Source: three-view drawing plus pictorial views. Frame: mm from the lowest corner of the part. A direction names the side the tool comes from. Coordinates: 2 decimals unless noted, no trailing zeros. Write each loop counter-clockwise with the first axis right and the second up, starting at its lowest first coordinate (ties: lowest second). Pieces come first, ordered by that corner, then holes. Notation, with made-up numbers: M 78,53 L 113,53 A21 ccw 113,74 Z; hole C 24,35.5 d9. An arc over 180 degrees is marked long. Use CSV: the item, a comma, the result in double quotes.
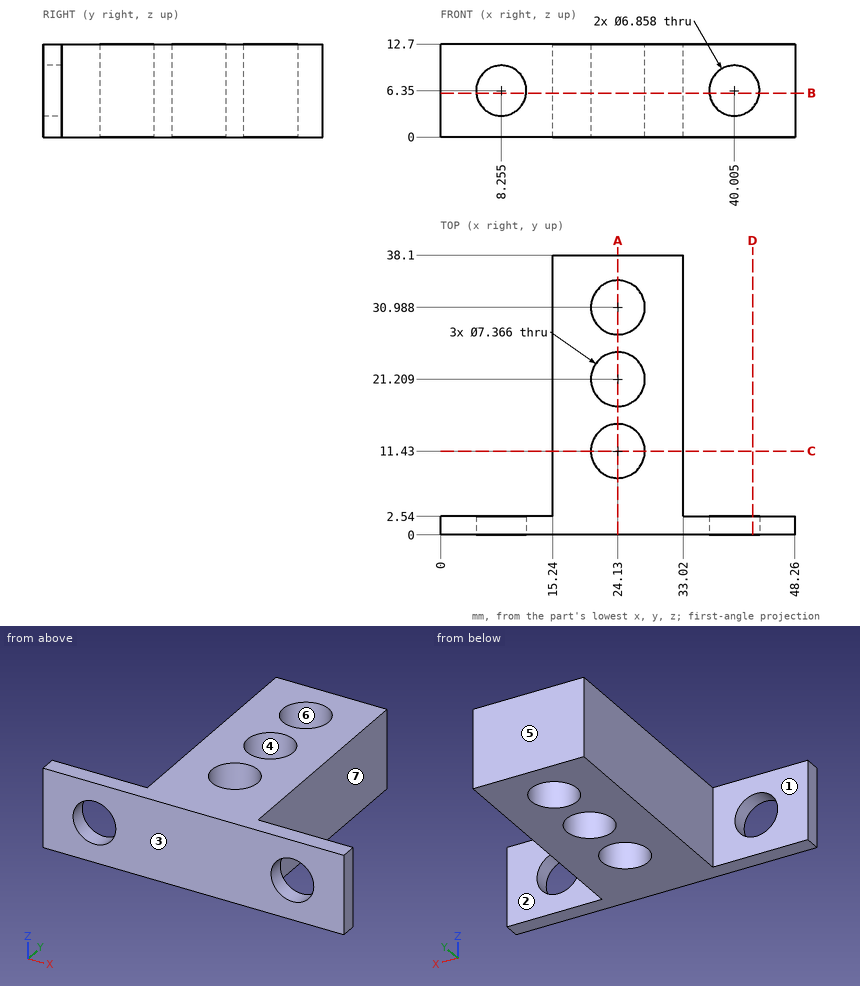
1. Section A-A (x = 24.13). Return loops of the section in (y, z) (3 decimals), then the cut area to 3 significant figures.
Resolved:
outline,"M 0,0 L 7.747,0 L 7.747,12.7 L 0,12.7 Z; M 15.113,0 L 17.526,0 L 17.526,12.7 L 15.113,12.7 Z; M 24.892,0 L 27.305,0 L 27.305,12.7 L 24.892,12.7 Z; M 34.671,0 L 38.1,0 L 38.1,12.7 L 34.671,12.7 Z"
area,"203 mm^2"
2. Access query for the marked faces 1, 2 and 3. Directions: +Z, -Z, +X, -X, +Y, -Y. A direction counts if a zero-diameter tool reaches every point of the face in a straight line with its end or side. Return the directions, or none.
Resolved:
face 1,"+Z, -Z, -X, +Y"
face 2,"+Z, -Z, +X, +Y"
face 3,"+Z, -Z, +X, -X, -Y"
3. Section B-B (z = 6). Return loops of the section in (x, y).
Resolved:
outline,"M 0,0 L 4.84,0 L 4.84,2.54 L 0,2.54 Z; M 11.67,0 L 36.59,0 L 36.59,2.54 L 33.02,2.54 L 33.02,38.1 L 15.24,38.1 L 15.24,2.54 L 11.67,2.54 Z; M 43.42,0 L 48.26,0 L 48.26,2.54 L 43.42,2.54 Z; hole C 24.13,11.43 d7.37; hole C 24.13,21.21 d7.37; hole C 24.13,30.99 d7.37"
4. Section C-C (y = 11.43). Return loops of the section in (x, z).
Resolved:
outline,"M 15.24,0 L 20.45,0 L 20.45,12.7 L 15.24,12.7 Z; M 27.81,0 L 33.02,0 L 33.02,12.7 L 27.81,12.7 Z"
5. Material intervals for line 1 (X direction, y = 1.7, z = 6.35); line 2 (Y direction, x = 24.13, z = 4.5) (3 decimals); line 3 (Y direction, x = 23, z = 5.25), sorted ascending. Write a range as [from, to].
Resolved:
line 1,"x = [0, 4.83], [11.68, 36.58], [43.43, 48.26]"
line 2,"y = [0, 7.747], [15.113, 17.526], [24.892, 27.305], [34.671, 38.1]"
line 3,"y = [0, 7.92], [14.94, 17.7], [24.71, 27.48], [34.49, 38.1]"
6. Section D-D (x = 42.5). Return loops of the section in (y, z).
Resolved:
outline,"M 0,0 L 2.54,0 L 2.54,4 L 0,4 Z; M 0,8.7 L 2.54,8.7 L 2.54,12.7 L 0,12.7 Z"
7. Mould query, pull axis Y, two halves, no side actions, for the marked faces 4, 5, 6 and 7. Classes: pulls with the +Y half, pulls with the -Y half, needs draft (parallel to the pull), parting line crosses it, or undercut.
Resolved:
face 4,"undercut"
face 5,"pulls with the +Y half"
face 6,"undercut"
face 7,"needs draft"
8. Contact query for flat-ended pins moving along their axis: pin 1 Ø4 at (x, z) = (35.5, 5) entering from +Y; pin 2 Ø6 at (x, y) = (24.13, 21.209) entering from -Z; pin 3 Ø6.5 at (y, z) = (27.5, 6.5) entering from -X. Output: stop coordinate, or through.
Resolved:
pin 1,"stops at y = 2.54"
pin 2,"passes through"
pin 3,"stops at x = 15.24"
